from build123d import *

# Parameters (mm, degrees)
SKETCH1_R           = 10.8
BOSS_EXTRUDE2_DEPTH = 6.35
FILLET1_R           = 35
SKETCH2_W           = 6.6
SKETCH2_H           = 6.6
CUT_EXTRUDE1_DEPTH  = 135.431204491


with BuildPart() as part:
    # Sketch1 → Boss-Extrude2 (new body)
    with BuildSketch(Plane.XY):
        Circle(SKETCH1_R)
        with BuildLine():
            ThreePointArc((-0.315151241, -1.312699393), (70.647078237, 42.17301076), (27.161368085, 113.135240238))
            ThreePointArc((27.161368085, 113.135240238), (25.533517451, 112.137692087), (26.531065602, 110.509841453))
            ThreePointArc((26.531065602, 110.509841453), (68.021679452, 42.803313242), (0.315151241, 1.312699393))
            ThreePointArc((0.315151241, 1.312699393), (-1.312699393, 0.315151241), (-0.315151241, -1.312699393))
        make_face()
    extrude(amount=BOSS_EXTRUDE2_DEPTH)

    # Fillet1
    fillet1_edges = [part.edges().sort_by_distance(p)[0] for p in [
        (10.798543624, -0.177357298, 3.175),
        (10.413952601, -2.861746185, 3.175),
    ]]
    fillet(fillet1_edges, radius=FILLET1_R)

    # Sketch2 → Cut-Extrude1 (cut, through all)
    with BuildSketch(Plane.XY.offset(6.35)):
        with Locations((0, -3.3)):
            Rectangle(SKETCH2_W, SKETCH2_H)
        Polygon((-5.6, 0), (-3.3, 0), (3.3, 0), (5.6, 0), (5.6, 5.2), (-5.6, 5.2), align=None)
    extrude(amount=-CUT_EXTRUDE1_DEPTH, mode=Mode.SUBTRACT)


solid = part.part
The model under review builds one solid part; all positions refer to its coordinate system, in mm. A direction names the side the tool comes from. Coordinates: 2 decimals unless noted, no trailing zeros. Loops run counter-clockwise (first coordinate to the right, second up) from the corner with the lowest first, then second, coordinate; pieces in that order, holes last. Notation, with made-up numbers: (-1, -34.75) -> (23, -34.75) arc R20 ccw to (23, -19.75) -> close; hole circle Ø5 at (-39, 39.5). An arc over 180 degrees is marked (long way). Use a Markdown table: item, result. Add a question column.
1. Add section C-C on y = 64.5. Write out the cut boundary in (x, z), plus the area to 3 significant figures.
2. To check wall thickness, follow line 1 (X direction, y = 55, z = 0.75); line 2 (X direction, y = 3, z = 1); line 3 (Y direction, x = 60, z = 1.75). State the ranges of each line that lie inside material, in increasing order.
3. Draft analysis for pull direction X (two halves, no side actions). For faces 1 (the face through (40, 6, 6.35)), 2 (the face through (0, 5.2, 3)), 3 (the face through (72.152, 52.139, 3.131)), state which applies: pulls with the +X half, pulls with the -X half, needs draft (parallel to the pull), parting line crosses it, or undercut.
4. Machinability: for faces 4 (the face through (40, 6, 0)), 5 (the face through (5.6, 3, 3)), which of the approach directions +Z, -Z, +X, -X, +Y, -Y give a long, thin tool a straight path to every point of the face, cutting with its end or side? Answer none if there is none.
5. Add section A-A on x = 0. Write out the cut boundary in (y, z), plus the area to 3 significant figures.
6. Add section B-B on y = 105. Write out the cut boundary in (x, z).
7. Clearance check with flat-ended pins moving along their axes: pin 1 Ø1.5 at (x, z) = (18, 5) entering from +Y; pin 2 Ø1.6 at (y, z) = (3.5, 2.5) entering from +X; pin 3 Ø2.5 at (y, z) = (4, 3.5) entering from -X. State where each tip first meets the part, or that it passes through.
Returned:
| question | item | result |
|---|---|---|
| 1 | outline | (68.91, 0) -> (71.64, 0) -> (71.64, 6.35) -> (68.91, 6.35) -> close |
| 1 | area | 17.3 mm² |
| 2 | line 1 | x = 69.57 to 72.27 |
| 2 | line 2 | x = -10.37 to -5.6, 5.6 to 39.19 |
| 2 | line 3 | y = 19.94 to 24.55, 87.27 to 91.88 |
| 3 | face 1 | needs draft |
| 3 | face 2 | undercut |
| 3 | face 3 | pulls with the +X half |
| 4 | face 4 | -Z, +X, -X, +Y, -Y |
| 4 | face 5 | +Z, -Z |
| 5 | outline | (-10.8, 0) -> (-6.6, 0) -> (-6.6, 6.35) -> (-10.8, 6.35) -> close; (5.2, 0) -> (10.8, 0) -> (10.8, 6.35) -> (5.2, 6.35) -> close |
| 5 | area | 62.2 mm² |
| 6 | outline | (40.68, 0) -> (45.88, 0) -> (45.88, 6.35) -> (40.68, 6.35) -> close |
| 7 | pin 1 | stops at y = 4.19 |
| 7 | pin 2 | stops at x = 41.7 |
| 7 | pin 3 | stops at x = -10.44 |
